Geometry: see drawing. Coordinates: mm, zero at the bounding-box minimum. Round coordinates to 2 decimals unless told otherwise and drop trailing zeros. Write each loop counter-clockwise with the first axis right and the second up, starting at its lowest first coordinate (ties: lowest second). Pieces come first, ordered by that corner, then holes. Notation, with made-up numbers: (-9.5, -37.5) -> (8.5, -37.5) arc R25 ccw to (8.5, -5.5) -> close; hole circle Ø1 at (24, 8). An arc over 180 degrees is marked (long way). Write item = value, one per line. Start each with the question number.
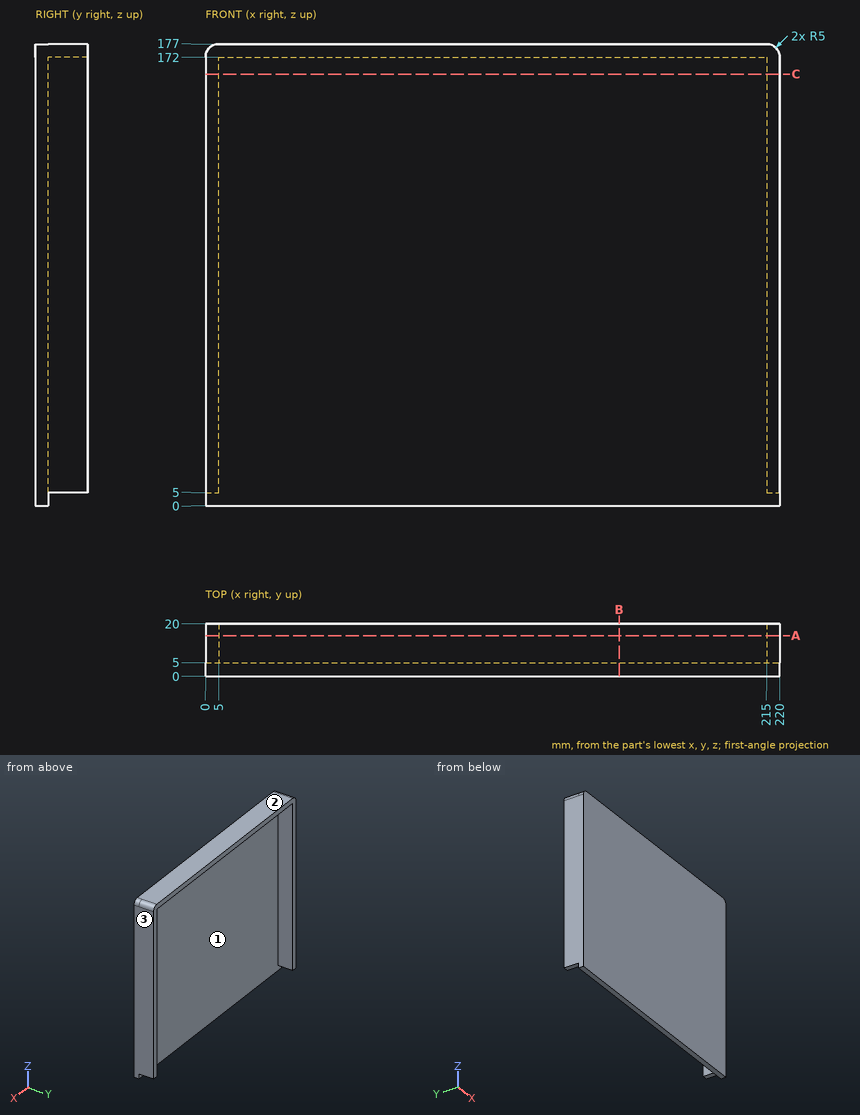
1. Pin query (flat end, axial travel): P1, Ø5, axis at x = 24.5, y = 10, coming from the -Z side; P2, Ø5.5, axis at x = 218, y = 11.5, coming from the -Z side; P3, Ø5, axis at x = 84.5, z = 23, coming from the +Y side. Return the tip coordinate at first contact, or that it passes through.
2. Line query: line 1 along X through (y, z) = (16, 85); line 2 along Y through (x, z) = (124, 142); line 3 along Z through (x, y) = (86.5, 7.5). Output: solid intervals per line, ascending.
3. Section B-B (x = 158.5). Output: boundary loops of the cut face in (y, z).
4. Section A-A (y = 15.5). Output: boundary loops of the cut face in (x, z).
5. Section C-C (z = 165.5). Output: boundary loops of the cut face in (x, y), then the cut area to 3 significant figures.
6. Mould query, pull axis X, two halves, no side actions, for the marked faces 1, 2 and 3. Classes: pulls with the +X half, pulls with the -X half, needs draft (parallel to the pull), parting line crosses it, or undercut.
Check sheet entries:
q1.P1 = 172
q1.P2 = 5
q1.P3 = 5
q2.line_1 = 0 to 5, 215 to 220
q2.line_2 = 0 to 5
q2.line_3 = 172 to 177
q3.outline = (0, 0) -> (5, 0) -> (5, 172) -> (20, 172) -> (20, 177) -> (0, 177) -> close
q4.outline = (0, 5) -> (5, 5) -> (5, 172) -> (215, 172) -> (215, 5) -> (220, 5) -> (220, 172) arc R5 ccw to (215, 177) -> (5, 177) arc R5 ccw to (0, 172) -> close
q5.outline = (0, 0) -> (220, 0) -> (220, 20) -> (215, 20) -> (215, 5) -> (5, 5) -> (5, 20) -> (0, 20) -> close
q5.area = 1,250 mm2
q6.face_1 = undercut
q6.face_2 = needs draft
q6.face_3 = pulls with the +X half
